Design review of the part built by this model. Coordinates are the model's own, in mm. Face numbers are marked on the shaded views. A direction names the side the tool comes from. Coordinates: 2 decimals unless noted, no trailing zeros. Write each loop counter-clockwise with the first axis right and the second up, starting at its lowest first coordinate (ties: lowest second). Pieces come first, ordered by that corner, then holes. Notation, with made-up numbers: (48, -9.75) -> (95, -9.75) arc R25 ccw to (95, 11.25) -> close; hole circle Ø1 at (-8.75, 16). An arc over 180 degrees is marked (long way). Answer in a Markdown table with one row per item. Add a question column.
Item 1: Take a section at B-B, the plane y = 25. Write out the cut boundary in (x, z), and give its area (3 significant figures).
Item 2: Draft analysis for pull direction X (two halves, no side actions). For the marked faces 1, 2 and 3, state which applies: released by +X, released by -X, zero draft, split by the parting line, or undercut.
Item 3: For the marked faces 4, 5 and 6, list the 3-axis set-ups (+Z, -Z, +X, -X, +Y, -Y) from which the entire face can be reached by the end or side of a thin tool; tool diameter is ignored.
Item 4: Clearance check with flat-ended pins moving along their axes: P1, Ø1, axis at x = 143, y = 56.5, coming from the -Z side; P2, Ø6, axis at y = 67.5, z = 19, coming from the +X side; P3, Ø6, axis at x = -22.5, y = 59.5, coming from the +Z side. State where each tip first meets the part, or that it passes through.
Item 5: Take a section at A-A, the plane x = -41.5. Write out the cut boundary in (y, z), and give its area (3 significant figures).
Item 6: Take a section at D-D, the plane y = 58.5. Write out the cut boundary in (x, z), and give its area (3 significant figures).
Item 7: To check wall thickness, follow line 1 (X direction, y = 36, z = -15); line 2 (Y direction, x = 111, z = -35); line 3 (X direction, y = 10.5, z = -26). State the ranges of each line that lie inside material, in increasing order.
Item 8: Take a section at C-C, the plane z = -26. Write out the cut boundary in (x, y), and give its area (3 significant figures).
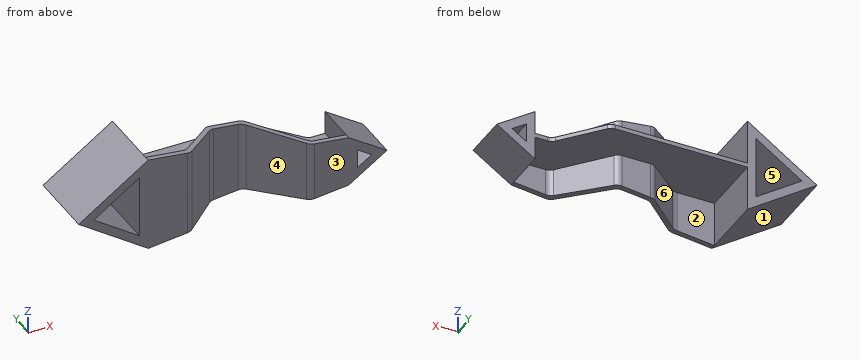
from build123d import *

# Parameters (mm, degrees)
BOSS_EXTRUDE1_DEPTH     = 82
BOSS_EXTRUDE2_DEPTH     = 56
BOSS_EXTRUDE3_START     = -25
BOSS_EXTRUDE3_DEPTH     = 54.666666667
BOSS_EXTRUDE4_DEPTH     = 2.5
CUT_EXTRUDE2_DEPTH      = 83
CUT_EXTRUDE2_DEPTH_BACK = 26
FILLET1_R               = 10


with BuildPart() as part:
    # Sketch2 → Boss-Extrude1 (new body)
    with BuildSketch(Plane(origin=(0, 0, 0), x_dir=(1, 0, 0), z_dir=(0, 1, 0))):
        Polygon((0, -56), (0, 56), (-82, 0), align=None)
        Polygon((-10, 37.0612765), (-64.268297732, 0), (-10, -37.0612765), align=None, mode=Mode.SUBTRACT)
    extrude(amount=BOSS_EXTRUDE1_DEPTH)

    # Sketch3 → Boss-Extrude2 (add, symmetric)
    with BuildSketch(Plane.XY):
        Polygon((0, 0), (50, 0), (91.711375741, 35), (128.654022129, 35), (179, -25), (224, -25), (224, -19), (181.797845949, -19), (131.451868078, 41), (89.527554335, 41), (47.816178594, 6), (0, 6), align=None)
    extrude(amount=BOSS_EXTRUDE2_DEPTH, both=True)

    # Sketch4 → Boss-Extrude3 (add)
    with BuildSketch(Plane(origin=(0, 0, 0), x_dir=(1, 0, 0), z_dir=(0, 1, 0)).offset(BOSS_EXTRUDE3_START)):
        Polygon((224, -30), (224, 30), (269, 0), align=None)
        Polygon((234, 11.314829082), (250.972243623, 0), (234, -11.314829082), align=None, mode=Mode.SUBTRACT)
    extrude(amount=BOSS_EXTRUDE3_DEPTH)

    # Sketch7 → Boss-Extrude4 (add, symmetric)
    with BuildSketch(Plane.XY):
        Polygon((0, 82), (160.578604614, 82), (204.491485312, 29.666666667), (224, 29.666666667), (224, -19), (181.797845949, -19), (131.451868078, 41), (89.527554335, 41), (47.816178594, 6), (0, 6), align=None)
    extrude(amount=BOSS_EXTRUDE4_DEPTH, both=True)

    # Sketch8 → Cut-Extrude2 (cut, two sides)
    with BuildSketch(Plane(origin=(0, 0, 0), x_dir=(1, 0, 0), z_dir=(0, 1, 0))) as cut_extrude2_sk:
        Polygon((0, 56), (224, 56), (224, 30), align=None)
        Polygon((0, -56), (224, -30), (224, -56), align=None)
    extrude(amount=CUT_EXTRUDE2_DEPTH, mode=Mode.SUBTRACT)
    extrude(cut_extrude2_sk.sketch, amount=-CUT_EXTRUDE2_DEPTH_BACK, mode=Mode.SUBTRACT)

    # Fillet1
    fillet1_edges = [part.edges().sort_by_distance(p)[0] for p in [
        (47.816178594, 6, 26.474953921),
        (89.527554335, 41, 24.054204436),
        (131.451868078, 41, 21.621096942),
        (181.797845949, -19, 18.699232155),
        (179, -25, 0),
        (128.654022129, 35, 0),
        (91.711375741, 35, 0),
        (50, 0, 0),
        (47.816178594, 6, -26.474953921),
        (89.527554335, 41, -24.054204436),
        (131.451868078, 41, -21.621096942),
        (181.797845949, -19, -18.699232155),
        (204.491485312, 29.666666667, 0),
        (160.578604614, 82, 0),
    ]]
    fillet(fillet1_edges, radius=FILLET1_R)


solid = part.part
Answers:
| question | item | result |
|---|---|---|
| 1 | outline | (-82, 0) -> (0, -56) -> (0, -2.5) -> (70.46, -2.5) -> (70.46, -47.82) -> (79.79, -46.74) -> (79.79, 46.74) -> (70.46, 47.82) -> (70.46, 2.5) -> (0, 2.5) -> (0, 56) -> close; (137.05, -40.09) -> (144.88, -39.18) -> (144.88, -2.5) -> (224, -2.5) -> (224, -30) -> (269, 0) -> (224, 30) -> (224, 2.5) -> (144.88, 2.5) -> (144.88, 39.18) -> (137.05, 40.09) -> close; hole (-64.27, 0) -> (-10, -37.06) -> (-10, 37.06) -> close; hole (234, -11.31) -> (250.97, 0) -> (234, 11.31) -> close |
| 1 | area | 5,990 mm^2 |
| 2 | face 1 | released by -X |
| 2 | face 2 | undercut |
| 2 | face 3 | zero draft |
| 3 | face 4 | +Z, -Z, -Y |
| 3 | face 5 | +Y, -Y |
| 3 | face 6 | -Z, +Y |
| 4 | P1 | stops at z = -2.5 |
| 4 | P2 | stops at x = 0 |
| 4 | P3 | stops at z = 42.68 |
| 5 | outline | (0, -27.66) -> (82, -27.66) -> (82, -15.55) -> (0, -15.55) -> close; (0, 15.55) -> (82, 15.55) -> (82, 27.66) -> (0, 27.66) -> close |
| 5 | area | 1,990 mm^2 |
| 6 | outline | (-82, 0) -> (0, -56) -> (0, -2.5) -> (180.3, -2.5) -> (180.3, 2.5) -> (0, 2.5) -> (0, 56) -> close; hole (-64.27, 0) -> (-10, -37.06) -> (-10, 37.06) -> close |
| 6 | area | 3,480 mm^2 |
| 7 | line 1 | x = -60.04 to -42.3, -10 to 0, 83.57 to 135.65 |
| 7 | line 2 | y = 35 to 41 |
| 7 | line 3 | x = -43.93 to -26.2, -10 to 0, 53.18 to 62.51, 149.21 to 157.04, 224 to 230 |
| 8 | outline | (-43.93, 0) -> (-26.2, 0) -> (-26.2, 82) -> (-43.93, 82) -> close; (-10, 0) -> (46.36, 0) arc R10 ccw to (52.79, 2.34) -> (88.92, 32.66) arc R10 cw to (95.35, 35) -> (123.99, 35) arc R10 cw to (131.65, 31.43) -> (176, -21.43) arc R10 ccw to (183.66, -25) -> (230, -25) -> (230, 29.67) -> (224, 29.67) -> (224, -19) -> (186.46, -19) arc R10 cw to (178.8, -15.43) -> (134.45, 37.43) arc R10 ccw to (126.79, 41) -> (93.17, 41) arc R10 ccw to (86.74, 38.66) -> (50.6, 8.34) arc R10 cw to (44.18, 6) -> (0, 6) -> (0, 82) -> (-10, 82) -> close |
| 8 | area | 4,190 mm^2 |
